Design review of the part shown in the three views and the two pictorial views. Dimensions are in mm from the part's minimum x, y and z. A direction names the side the tool comes from. Round coordinates to 2 decimals unless told otherwise and drop trailing zeros. Order: outer loops, then holes, each group sorted by start corner. A loop starts at its lowest first (then second) coordinate and runs counter-clockwise, first axis right, second up.
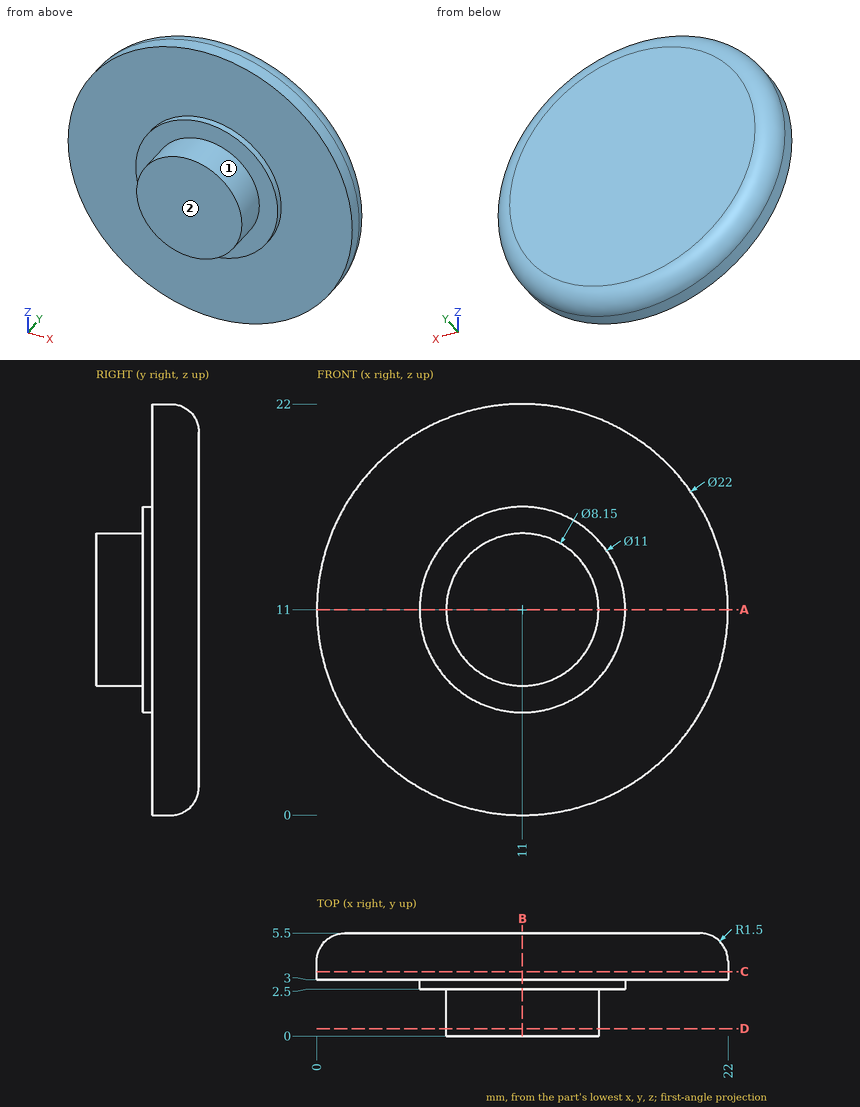
1) Take a section at D-D on y = 0.4. Give the boundary of the cut face in (x, z) (3 decimals), plus the area to 3 significant figures.
Results:
outline: circle Ø8.15 at (11, 11)
area: 52.2 mm2
2) Take a section at B-B on x = 11. Give the boundary of the cut face in (y, z) (3 decimals).
Results:
outline: (0, 6.925) - (2.5, 6.925) - (2.5, 5.5) - (3, 5.5) - (3, 0) - (4, 0) arc R1.5 ccw to (5.5, 1.5) - (5.5, 20.5) arc R1.5 ccw to (4, 22) - (3, 22) - (3, 16.5) - (2.5, 16.5) - (2.5, 15.075) - (0, 15.075) - close
3) Take a section at C-C on y = 3.45. Give the boundary of the cut face in (x, z), plus the area to 3 significant figures.
Results:
outline: circle Ø22 at (11, 11)
area: 380 mm2
4) Clearance check with a flat-ended pin moving along its axis: P1, Ø4, axis at x = 19, z = 14, coming from the -Y side. State where the tip first meets the part, or that it passes through.
Results:
P1: stops at y = 3
5) For the marked faces 1 and 2, list the 3-axis set-ups (+Z, -Z, +X, -X, +Y, -Y) from which the entire face can be reached by the end or side of a thin tool; tool diameter is ignored.
Results:
face 1: -Y
face 2: +Z, -Z, +X, -X, -Y
6) To check wall thickness, follow line 1 along Y through (x, z) = (15.75, 9); line 2 along Y through (x, z) = (18.5, 6.25); line 3 along Z through (x, y) = (14, 3.1). State the ranges of each line that lie inside material, in increasing order.
Results:
line 1: y = 2.5 to 5.5
line 2: y = 3 to 5.5
line 3: z = 0.42 to 21.58
7) Take a section at A-A on z = 11. Give the boundary of the cut face in (x, y) (3 decimals).
Results:
outline: (0, 3) - (5.5, 3) - (5.5, 2.5) - (6.925, 2.5) - (6.925, 0) - (15.075, 0) - (15.075, 2.5) - (16.5, 2.5) - (16.5, 3) - (22, 3) - (22, 4) arc R1.5 ccw to (20.5, 5.5) - (1.5, 5.5) arc R1.5 ccw to (0, 4) - close
